Design review of the part built by this model. Coordinates are the model's own, in mm. Face numbers are marked on the shaded views. A direction names the side the tool comes from. Coordinates: 2 decimals unless noted, no trailing zeros. Order: outer loops, then holes, each group sorted by start corner. A loop starts at its lowest first (then second) coordinate and runs counter-clockwise, first axis right, second up. Notation, with made-up numbers: (38.25, 44) -> (85.25, 44) arc R19 ccw to (85.25, 72) -> close; hole circle Ø7 at (-38.75, 84). An arc over 180 degrees is marked (long way). Write item = value, one per line.
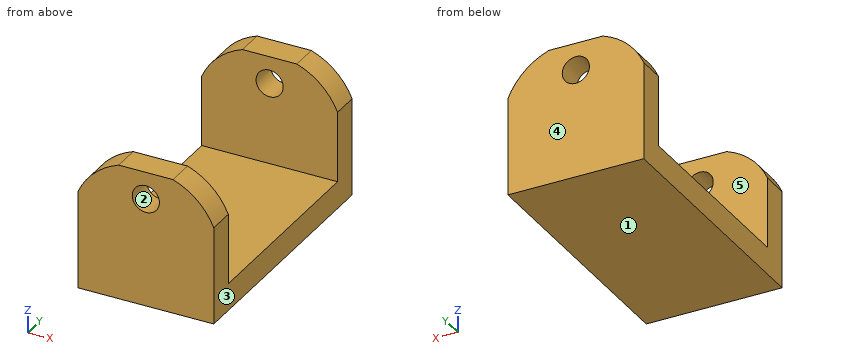
```python
from build123d import *

# Parameters (mm, degrees)
SKETCH1_R           = 2.5
BOSS_EXTRUDE1_DEPTH = 47.65
SKETCH2_W           = 20
SKETCH2_H           = 37.65
CUT_EXTRUDE1_DEPTH  = 60.333991101


with BuildPart() as part:
    # Sketch1 → Boss-Extrude1 (new body)
    with BuildSketch(Plane(origin=(0, 0, 0), x_dir=(1, 0, 0), z_dir=(0, 1, 0))):
        with BuildLine():
            Line((-5, 0), (5, 0))
            ThreePointArc((5, 0), (9.487755282, 2.709547912), (12.5, 7))
            Line((12.5, 7), (12.5, 25))
            Line((12.5, 25), (-12.5, 25))
            Line((-12.5, 25), (-12.5, 7))
            ThreePointArc((-12.5, 7), (-9.487755282, 2.709547912), (-5, 0))
        make_face()
        with Locations(Location((0, 5, 0), (0, 0, 270))):
            Circle(SKETCH1_R, mode=Mode.SUBTRACT)
    extrude(amount=BOSS_EXTRUDE1_DEPTH)

    # Sketch2 → Cut-Extrude1 (cut, through all)
    with BuildSketch(Plane.ZY.offset(12.5)):
        with Locations((-10, 23.825)):
            Rectangle(SKETCH2_W, SKETCH2_H)
    extrude(amount=-CUT_EXTRUDE1_DEPTH, mode=Mode.SUBTRACT)


solid = part.part
```
(1) For the marked faces 4 and 5, list the 3-axis set-ups (+Z, -Z, +X, -X, +Y, -Y) from which the entire face can be reached by the end or side of a thin tool; tool diameter is ignored.
Report:
face_4 = +Z, -Z, +X, -X, +Y
face_5 = +Z, +X, -X
(2) The part is to be moulded in two halves that separate along X. For the marked faces 1, 2 and 3, say which applies: released by +X, released by -X, zero draft, split by the parting line, or undercut.
Report:
face_1 = zero draft
face_2 = undercut
face_3 = released by +X
(3) We need section D-D (z = -5). Write out the cut boundary in (x, y).
Report:
outline = (-11.42, 0) -> (-2.5, 0) -> (-2.5, 5) -> (-11.42, 5) -> close; (-11.42, 42.65) -> (-2.5, 42.65) -> (-2.5, 47.65) -> (-11.42, 47.65) -> close; (2.5, 0) -> (11.42, 0) -> (11.42, 5) -> (2.5, 5) -> close; (2.5, 42.65) -> (11.42, 42.65) -> (11.42, 47.65) -> (2.5, 47.65) -> close
(4) Insertion check: pin 1 (1 mm diameter, centred on x = 5.5, y = 18, fed in from +Z); pin 2 (4.5 mm diameter, centred on x = 0, z = -5, fed in from +Y). Each pin has a flat end and moves straight along its axis. Give the tip position at first contact, or say it passes through.
Report:
pin_1 = -20
pin_2 = through
(5) We need section C-C (x = 4). Write out the cut boundary in (y, z).
Report:
outline = (0, -25) -> (47.65, -25) -> (47.65, 0) -> (42.65, 0) -> (42.65, -20) -> (5, -20) -> (5, 0) -> (0, 0) -> close
(6) We need section B-B (x = 0). Write out the cut boundary in (y, z).
Report:
outline = (0, -25) -> (47.65, -25) -> (47.65, -7.5) -> (42.65, -7.5) -> (42.65, -20) -> (5, -20) -> (5, -7.5) -> (0, -7.5) -> close; (0, -2.5) -> (5, -2.5) -> (5, 0) -> (0, 0) -> close; (42.65, -2.5) -> (47.65, -2.5) -> (47.65, 0) -> (42.65, 0) -> close
(7) For L1, parallel to Y at x = 8.5, z = -2.5; L2, parallel to Z at x = 0, y = 46.3; L3, parallel to Z at x = -9, y = 30, list the stretches that pass through material, from the lowest coordinate up.
Report:
L1 = 0 to 5, 42.65 to 47.65
L2 = -25 to -7.5, -2.5 to 0
L3 = -25 to -20
(8) We need section A-A (z = -12). Write out the cut boundary in (x, y), and give its area (3 significant figures).
Report:
outline = (-12.5, 0) -> (12.5, 0) -> (12.5, 5) -> (-12.5, 5) -> close; (-12.5, 42.65) -> (12.5, 42.65) -> (12.5, 47.65) -> (-12.5, 47.65) -> close
area = 250 mm²
